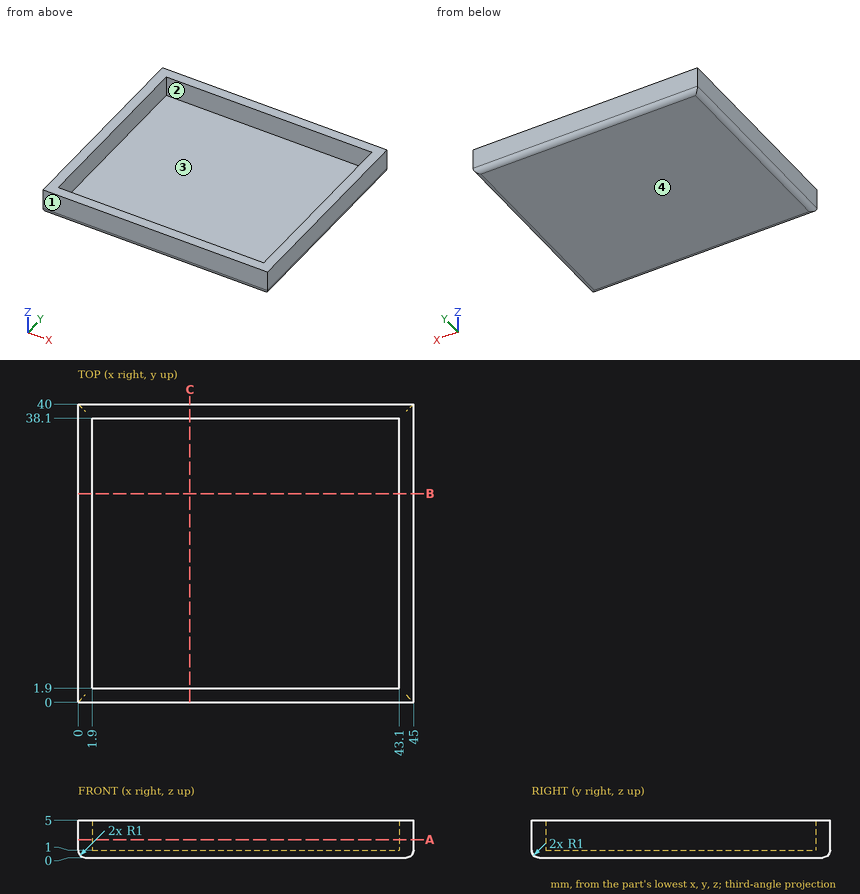
Job drawing, mm, ordinate dimensions from the low corner. One solid piece. A direction names the side the tool comes from. Coordinates: 2 decimals unless noted, no trailing zeros. Write each loop counter-clockwise with the first axis right and the second up, starting at its lowest first coordinate (ties: lowest second). Pieces come first, ordered by that corner, then holes.
Item 1: Probe line 1 (X direction, y = 11.5, z = 3.05); line 2 (Y direction, x = 28, z = 1.1); line 3 (Z direction, x = 34.5, y = 22). List the from-to ranges inside material, lowest first.
Item 2: Mould opens along X. For the marked faces 3 and 4 say: released by +X, released by -X, zero draft, split by the parting line, or undercut.
Item 3: Pin check, flat tip, straight feed: pin 1 (3 mm diameter, centred on x = 5.5, y = 24.5, fed in from +Z). Stop position of the tip, or through.
Item 4: Slice it at A-A (z = 2.4). Write the cut outline in (x, y), and give its area (3 significant figures).
Item 5: Which spindle directions (+Z, -Z, +X, -X, +Y, -Y) get a long thin tool onto all of the face, cutting with end or side? Do the marked faces 1 and 2. Say none if no direction does.
Item 6: Slice it at B-B (y = 28). Write the cut outline in (x, z), and give its area (3 significant figures).
Item 7: Slice it at C-C (x = 15). Write the cut outline in (y, z), and give its area (3 significant figures).
Results found:
1. line 1: x = 0 to 1.9, 43.1 to 45
1. line 2: y = 0 to 1.9, 38.1 to 40
1. line 3: z = 0 to 1
2. face 3: undercut
2. face 4: zero draft
3. pin 1: stops at z = 1
4. outline: (0, 0) - (45, 0) - (45, 40) - (0, 40) - close; hole (1.9, 1.9) - (43.1, 1.9) - (43.1, 38.1) - (1.9, 38.1) - close
4. area: 309 mm2
5. face 1: +Z, -Z, +X, -X, -Y
5. face 2: +Z
6. outline: (0, 1) arc R1 ccw to (1, 0) - (44, 0) arc R1 ccw to (45, 1) - (45, 5) - (43.1, 5) - (43.1, 1) - (1.9, 1) - (1.9, 5) - (0, 5) - close
6. area: 59.8 mm2
7. outline: (0, 1) arc R1 ccw to (1, 0) - (39, 0) arc R1 ccw to (40, 1) - (40, 5) - (38.1, 5) - (38.1, 1) - (1.9, 1) - (1.9, 5) - (0, 5) - close
7. area: 54.8 mm2
